Part model, mm, in its own coordinate system. A direction names the side the tool comes from. Give positions to 0.01 mm unless a question says otherwise; leave off trailing zeros. Order: outer loops, then holes, each group sorted by start corner. A loop starts at its lowest first (then second) coordinate and runs counter-clockwise, first axis right, second up. Notation, with made-up numbers: (18, -9) - (43, -9) arc R28 ccw to (43, 25) - close; hole circle Ø1 at (36, -5.75). An arc over 180 degrees is marked (long way). One line per item, written item: value.
```python
from build123d import *


with BuildPart() as f2:
    # F2: sweep along a path in F1
    with BuildLine(Plane.YZ) as f2_path:
        Line((0, 0), (0, 710))
        Line((0, 710), (710, 710))
        Line((710, 710), (710, 0))
        Line((710, 0), (0, 0))
    # F0 (on Top) → F2 (sweep)
    with BuildSketch(Plane.XY):
        Polygon((0, -15), (0, 0), (-40, 0), (-40, -15), (-38.5, -15), (-38.5, -1.5), (-1.5, -1.5), (-1.5, -15), align=None)
    sweep(path=f2_path.line, transition=Transition.RIGHT)


solid = f2.part
```
1) Which spindle directions (+Z, -Z, +X, -X, +Y, -Y) get a long thin tool onto all of the face, cutting with end or side? Do faces 1 (the flat face through (-20, 711.5, 350)), 2 (the flat face through (-20, 350, 0)), 3 (the flat face through (-40, 713, 521)), 4 (the flat face through (-20, 360, 711.5)). Say none if no direction does.
Outcome:
face 1: +Z, -Z, +Y
face 2: +X, -X
face 3: +Z, -Z, -X, +Y, -Y
face 4: +Z, +Y, -Y
2) Cut at A-A, the plane y = 189. Give the cut face in (x, z).
Outcome:
outline: (-40, -15) - (-38.5, -15) - (-38.5, -1.5) - (-1.5, -1.5) - (-1.5, -15) - (0, -15) - (0, 0) - (-40, 0) - close; (-40, 710) - (0, 710) - (0, 725) - (-1.5, 725) - (-1.5, 711.5) - (-38.5, 711.5) - (-38.5, 725) - (-40, 725) - close
3) Pin check, flat tips, straight feed: pin 1 (18.5 mm diameter, centred on x = -20, y = 391, fed in from -Z); pin 2 (12 mm diameter, centred on x = -14.5, y = 437.5, fed in from +Z); pin 3 (12 mm diameter, centred on x = -20.5, z = 76, fed in from +Y). Stop position of each tip, or through.
Outcome:
pin 1: stops at z = -1.5
pin 2: stops at z = 711.5
pin 3: stops at y = 711.5
4) Mould opens along Y. For faces 5 (the flat face through (-20, 360, 710)), 6 (the flat face through (-20, 350, -1.5)), 7 (the flat face through (-20, -1.5, 360)), 8 (the flat face through (-20, 710, 350)) say: released by +Y, released by -Y, zero draft, split by the parting line, or undercut.
Outcome:
face 5: undercut
face 6: zero draft
face 7: released by -Y
face 8: undercut
5) Cut at B-B, the plane x = -31. Give the cut face in (y, z), then the cut area to 3 significant figures.
Outcome:
outline: (-1.5, -1.5) - (711.5, -1.5) - (711.5, 711.5) - (-1.5, 711.5) - close; hole (0, 0) - (710, 0) - (710, 710) - (0, 710) - close
area: 4,270 mm^2
6) Drill centre line: line 1 along Y through (x, z) = (-25.5, 398). Where is it in solid material? Low to high. Write a range as from..to.
Outcome:
line 1: y = -1.5..0, 710..711.5
